Autodesk Inventor part; units mm, degrees
ref_plane "YZ Plane" through (0, 0, 0) normal (1, 0, 0) x (0, 1, 0)
ref_plane "XZ Plane" through (0, 0, 0) normal (0, 1, 0) x (-1, 0, 0)
ref_plane "XY Plane" through (0, 0, 0) normal (0, 0, 1) x (1, 0, 0)
sketch "Sketch1" plane through (0, 0, 0) normal (0, 0, 1) x (1, 0, 0)
  line L0 (3.175, 0) -> (28.575, 0)
  line L1 (31.75, 3.175) -> (31.75, 28.575)
  line L2 (0, 28.575) -> (0, 3.175)
  line L3 (4.7625, 3.175) -> (26.9875, 3.175)
  line L4 (28.575, 4.7625) -> (28.575, 28.575)
  line L5 (3.175, 28.575) -> (3.175, 4.7625)
  line L6 (0, 28.575) -> (3.175, 28.575)
  line L7 (28.575, 28.575) -> (31.75, 28.575)
  arc A0 (3.175, 4.7625) -> (4.7625, 3.175) centre (4.7625, 4.7625) ccw
  arc A1 (26.9875, 3.175) -> (28.575, 4.7625) centre (26.9875, 4.7625) ccw
  arc A2 (0, 3.175) -> (3.175, 0) centre (3.175, 3.175) ccw
  arc A3 (28.575, 0) -> (31.75, 3.175) centre (28.575, 3.175) ccw
  point P0 (0, 0)
  point P1 (0, 0)
  point P2 (31.75, 0)
  dimension "d0" = 31.75
  dimension "d1" = 28.575
  dimension "d2" = 1.5875
  dimension "d3" = 3.175
extrude "Extrusion1" add sketch "Sketch1" along normal blind 152.4
sketch "Sketch2" plane through (31.75, 3.175, 0) normal (1, 0, 0) x (0, 0, -1)
  line L0 (-152.4, 0) -> (-152.4, 25.4)
  line L1 (0, 0) -> (-152.4, 0)
  line L2 (-152.4, 12.7) -> (-139.7, 12.7)
  point P0 (0, -3.175)
  dimension "d6" = 12.7
sketch "Sketch3" plane through (3.175, 0, 0) normal (0, -1, 0) x (1, 0, 0)
  line L0 (0, 152.4) -> (25.4, 152.4)
  line L1 (0, 0) -> (0, 152.4)
  line L2 (12.7, 152.4) -> (12.7, 139.7)
  point P0 (-3.175, 0)
  dimension "d7" = 12.7
hole "Hole1" at (31.75, 15.875, 139.7) direction (-1, 0, 0) diameter 6.35 end through all
hole "Hole2" at (15.875, 0, 139.7) direction (0, 1, 0) diameter 6.35 end through all
pattern_linear "Rectangular Pattern1" count 6 spacing 25.4 along (0, 0, -1) of "Hole1", "Hole2"
properties part number "6 in bar"
Input: part model. Units: mm. Frame: model coordinates. A direction names the side the tool comes from. Round coordinates to 2 decimals unless told otherwise and drop trailing zeros. Loops run counter-clockwise (first coordinate to the right, second up) from the corner with the lowest first, then second, coordinate; pieces in that order, holes last. Notation, with made-up numbers: (16, 33) -> (61, 33) arc R18 ccw to (61, 49) -> close; hole circle Ø8 at (25, 63.5). An arc over 180 degrees is marked (long way). Use one line per item in the form item = value. Start each with the question number.
Item 1: Set-up query: faces 1 (the face through (30.14, 15.735, 92.072)), 2 (the face through (3.175, 17, 75)). Return all of +Z, -Z, +X, -X, +Y, -Y with unobstructed straight access to the full face (end or side cutting, diameter ignored); none if empty.
Item 2: Material intervals for L1, parallel to X at y = 9.25, z = 133 (3 decimals); L2, parallel to Y at x = 19.5, z = 53.5 (3 decimals); L3, parallel to Y at x = 3, z = 70.5 (3 decimals), sorted ascending. Write a range as from..to.
Item 3: Contact query for a flat-ended pin moving along its axis: pin 1 Ø7.5 at (x, z) = (15.875, 38.1) entering from +Y (3 decimals). Output: stop coordinate, or through.
Item 4: Section query C-C on x = 21.5. Return the cut outline in (y, z) (3 decimals).
Item 5: Section query A-A on z = 38.1. Count the separate pieces of the cut face and the enclosed holes in it, then the cut area to 3 significant figures.
Item 6: Mould query, pull axis Z, two halves, no side actions, for faces 3 (the face through (14.92, 1.61, 9.67)), 4 (the face through (16, 3, 0)), 5 (the face through (16, 3.175, 75)). Classes: pulls with the +Z half, pulls with the -Z half, needs draft (parallel to the pull), parting line crosses it, or undercut.
Ans:
q1.face_1 = +X, -X
q1.face_2 = +Z, -Z, +Y
q2.L1 = 0..3.175, 28.575..31.75
q2.L2 = 0..3.175
q2.L3 = 0.005..28.575
q3.pin_1 = 3.175
q4.outline = (0, 0) -> (3.175, 0) -> (3.175, 152.4) -> (0, 152.4) -> close
q5.separate_pieces = 4
q5.enclosed_holes = 0
q5.area = 198 mm^2
q6.face_3 = undercut
q6.face_4 = pulls with the -Z half
q6.face_5 = needs draft
